The model under review builds one solid part; all positions refer to its coordinate system, in mm. Coordinates: 2 decimals unless noted, no trailing zeros.
```python
from build123d import *

# Parameters (mm, degrees)
SKETCH1_W             = 145.55
SKETCH1_H             = 12.7
BOSS_EXTRUDE1_DEPTH   = 3.175
F_4_40_TAPPED_HOLE1_D = 2.2606
LPATTERN1_COUNT       = 5
LPATTERN1_PITCH       = 25.4
FILLET1_R             = 1


with BuildPart() as part:
    # Sketch1 → Boss-Extrude1 (new body)
    with BuildSketch(Plane.XY):
        Rectangle(SKETCH1_W, SKETCH1_H)
    extrude(amount=BOSS_EXTRUDE1_DEPTH)

    # #4-40 Tapped Hole1 (through all)
    with Locations(Plane(origin=(-50.8, 3.35, 3.175), x_dir=(1, 0, 0), z_dir=(0, 0, 1))):
        with Locations((0, 0), (0, -6.7)):
            f_4_40_tapped_hole1 = Hole(F_4_40_TAPPED_HOLE1_D / 2)

    # LPattern1: #4-40 Tapped Hole1 ×5
    with Locations(*[(i * LPATTERN1_PITCH, 0, 0) for i in range(1, LPATTERN1_COUNT)]):
        add(f_4_40_tapped_hole1, mode=Mode.SUBTRACT)

    # Fillet1
    fillet1_edges = [part.edges().sort_by_distance(p)[0] for p in [
        (-72.775, 6.35, 1.5875),
        (72.775, 6.35, 1.5875),
        (72.775, -6.35, 1.5875),
        (-72.775, -6.35, 1.5875),
    ]]
    fillet(fillet1_edges, radius=FILLET1_R)


solid = part.part
```
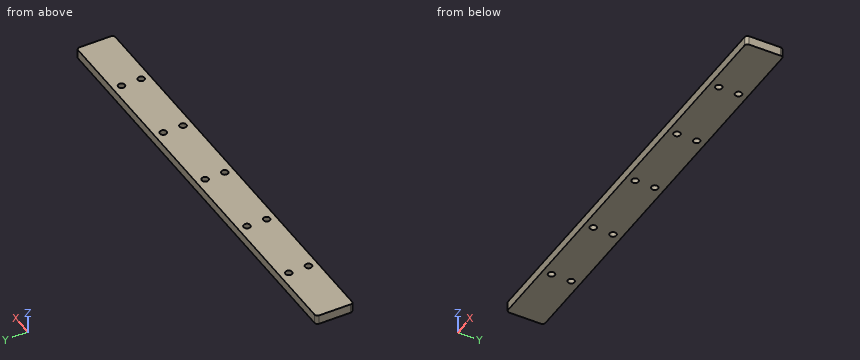
Item 1: For pin 1 (1.4 mm diameter, centred on x = 50.8, y = -3.35, fed in from +Z), flat-tipped, find the tip position at first contact; note if it passes through.
Solved:
pin 1: passes through
Item 2: To check wall thickness, follow line 1 along Y through (x, z) = (0, 0.6); line 2 along X through (y, z) = (-3, 2.4) (3 decimals); line 3 along X through (y, z) = (2.5, 0.9) (3 decimals). State the ranges of each line that lie inside material, in increasing order.
Solved:
line 1: y = -6.35 to -4.48, -2.22 to 2.22, 4.48 to 6.35
line 2: x = -72.775 to -51.875, -49.725 to -26.475, -24.325 to -1.075, 1.075 to 24.325, 26.475 to 49.725, 51.875 to 72.775
line 3: x = -72.775 to -51.545, -50.055 to -26.145, -24.655 to -0.745, 0.745 to 24.655, 26.145 to 50.055, 51.545 to 72.775
Item 3: Take a section at A-A, the plane z = 1.3. Count the separate pieces of the cut face and the enclosed holes in it, plus the area to 3 significant figures.
Solved:
separate pieces: 1
enclosed holes: 10
area: 1,810 mm2
